```python
from build123d import *

# Parameters (mm, degrees)
CUT_EXTRUDE_1_DEPTH = 3.5


with BuildPart() as part:
    # 草图1 → 旋转1 (revolve)
    with BuildSketch(Plane.XY):
        Polygon((-190, 25), (190, 25), (190, 11), (205, 11), (205, 10), (245, 10), (245, 8), (285, 8), (285, 0), (-235, 0), (-235, 8.5), (-205, 8.5), (-205, 11), (-190, 11), align=None)
    revolve(axis=Axis((-235, 0, 0), (1, 0, 0)))

    # 草图3 → 切除-拉伸1 (cut)
    with BuildSketch(Plane(origin=(0, -8, 0), x_dir=(-1, 0, 0), z_dir=(0, -1, 0))):
        with BuildLine():
            Line((-280, 3), (-250, 3))
            ThreePointArc((-250, 3), (-247, 0), (-250, -3))
            Line((-250, -3), (-280, -3))
            ThreePointArc((-280, -3), (-283, 0), (-280, 3))
        make_face()
    extrude(amount=-CUT_EXTRUDE_1_DEPTH, mode=Mode.SUBTRACT)


solid = part.part
```
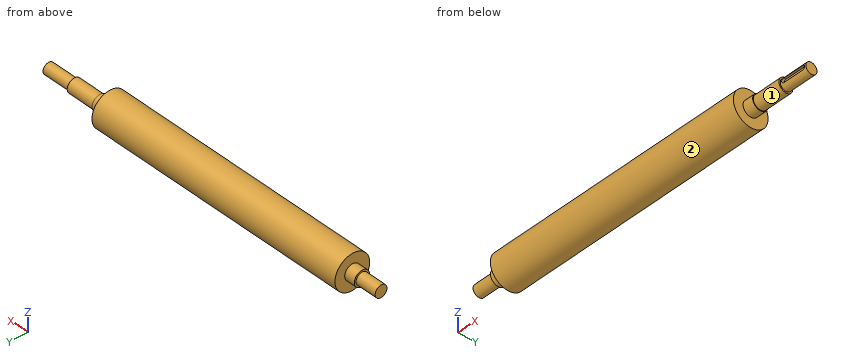
Work out the finished part from the listing and answer in its coordinate system (mm). Face numbers are marked on the shaded views. A direction names the side the tool comes from. Coordinates: 2 decimals unless noted, no trailing zeros. Write each loop counter-clockwise with the first axis right and the second up, starting at its lowest first coordinate (ties: lowest second). Pieces come first, ordered by that corner, then holes.
Q1. A cutting plane is placed at A-A, the plane y = 0.5. Give the vertices of the cut face in (x, z) (1 decimal).
Q2. Which of the six approach directions +Z, -Z, +X, -X, +Y, -Y give full straight-line access (tool end or side, diameter ignored) to the marked faces 1 and 2?
Q3. A cutting plane is placed at B-B, the plane z = -20. Give the vertices of the cut face in (x, y).
Q4. Find the intervals of material crossed by line 1 (X direction, y = 3, z = 12.5); line 2 (Z direction, x = -78, y = 2); line 3 (X direction, y = 8, z = -7), in increasing order.
Q5. Each of these flat-tipped pins is pushed along its axis until it touches: pin 1 Ø3 at (x, y) = (-112.5, -11.5) entering from +Z; pin 2 Ø3 at (y, z) = (4.5, -9.5) entering from -X; pin 3 Ø12 at (y, z) = (-10.5, 13) entering from +X. Where does it stop, or does it pass through?
Q6. A cutting plane is placed at D-D, the plane x = 198. Give the vertices of the cut face in (y, z), then the cut area to 3 significant figures.
Q7. A cutting plane is placed at C-C, the plane x = -114. Give the vertices of the cut face in (y, z), then the cut area to 3 significant figures.
Findings below:
1. outline: (-235, -8.5) - (-205, -8.5) - (-205, -11) - (-190, -11) - (-190, -25) - (190, -25) - (190, -11) - (205, -11) - (205, -10) - (245, -10) - (245, -8) - (285, -8) - (285, 8) - (245, 8) - (245, 10) - (205, 10) - (205, 11) - (190, 11) - (190, 25) - (-190, 25) - (-190, 11) - (-205, 11) - (-205, 8.5) - (-235, 8.5) - close
2. face 1: +X
2. face 2: +X, -X
3. outline: (-190, -15) - (190, -15) - (190, 15) - (-190, 15) - close
4. line 1: x = -190 to 190
4. line 2: z = -24.92 to 24.92
4. line 3: x = -205 to 205
5. pin 1: stops at z = 22.91
5. pin 2: stops at x = -205
5. pin 3: stops at x = 205
6. outline: circle Ø22 at (0, 0)
6. area: 380 mm2
7. outline: circle Ø50 at (0, 0)
7. area: 1,960 mm2
